Can you work these out from the model? Positions are in its coordinate system, mm. Face numbers are marked on the shaded views. A direction names the side the tool comes from. Give positions to 0.01 mm unless a question says otherwise; leave off trailing zeros. Order: outer loops, then holes, each group sorted by start corner. A loop starts at its lowest first (then second) coordinate and runs counter-clockwise, first axis right, second up. Notation, with made-up numbers: M 63,38.5 L 111,38.5 A33 cw 111,70.5 Z; hole C -28.75,60.25 d3. An arc over 180 degrees is marked long. One line per question, with ' | ' between items. Start each with the question number.
1) Please list where these lines run through material, in increasing order: line 1 along X through (y, z) = (0, 1.25); line 2 along Z through (x, y) = (-3.5, -4); line 3 along Y through (x, z) = (-11.5, -16.5). Write a range as [from, to].
2) For the marked faces 1 and 2, which set-ups out of +Z, -Z, +X, -X, +Y, -Y let a thin tool reach every point of the face, with its end or its side?
3) If we section it at A-A, the plane x = -9: Please give me the cut outline in (y, z).
4) If we section it at B-B, the plane y = 0: Please give me the cut outline in (x, z), plus the area to 3 significant figures.
5) If we section it at C-C, the plane z = -15.25: Please give me the cut outline in (x, y).
6) I'm going to push flat-ended pins straight in: pin 1 Ø1 at (x, y) = (8.5, -4.5) entering from -Z; pin 2 Ø8 at (x, z) = (0, -14.4) entering from -Y. Where does each tip first touch, or does it pass through?
7) If we section it at D-D, the plane x = 0: Please give me the cut outline in (y, z).
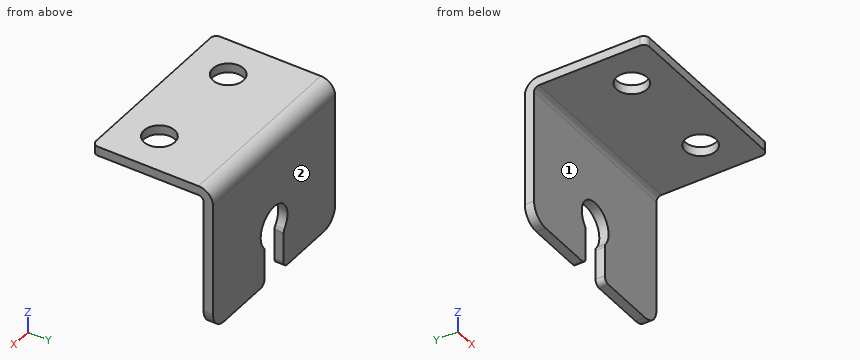
Autodesk Inventor part; units mm, degrees
ref_plane "YZ Plane" through (0, 0, 0) normal (1, 0, 0) x (0, 1, 0)
ref_plane "XZ Plane" through (0, 0, 0) normal (0, 1, 0) x (-1, 0, 0)
ref_plane "XY Plane" through (0, 0, 0) normal (0, 0, 1) x (1, 0, 0)
sketch "Sketch1" plane through (0, 0, 0) normal (0, 0, 1) x (1, 0, 0)
  line L0 (16, -7) -> (-16, -7)
  line L1 (-16, -7) -> (-16, 7)
  line L2 (-16, 7) -> (16, 7)
  line L3 (16, 7) -> (16, -7)
  line L4 (16, -7) -> (-16, 7) construction
  line L5 (-16, -7) -> (16, 7) construction
  line L6 (-9, 0) -> (9, 0) construction
  line L7 (-16, 7) -> (16, 7)
  line L8 (16, 7) -> (16, 12.25)
  line L9 (16, 12.25) -> (-16, 12.25)
  line L10 (-16, 12.25) -> (-16, 7)
  point P0 (0, 0)
  dimension "d126" = 32
  dimension "d127" = 14
  dimension "d128" = 7
  dimension "d129" = 12.25
extrude "Plate4" add sketch "Sketch1" along normal blind 1.6002
fillet "Fillet7" radius 1 2 edges at (16, -7, 0.8001) (-16, -7, 0.8001)
hole "Hole4" at (-9, 0, 0) at (9, 0, 0) direction (0, 0, 1) diameter 5.3 end through all
sketch "Sketch10" plane through (16, 12.25, 0) normal (0, 1, 0) x (-1, 0, 0)
  line L0 (32, 0) -> (0, 0)
  line L1 (0, 0) -> (0, -23.3998)
  line L2 (0, -23.3998) -> (32, -23.3998)
  line L3 (32, -23.3998) -> (32, 0)
edge flange "Flange5" height 25 angle 90 thickness 1.6002 bend radius 0.889 thickness toward (0, 1, 0) relief tear relief width 1.6002 relief depth 0.8001 edges at (0, 12.25, 0) wall of the first edge with corners at (-16, 12.25, 0) (16, 12.25, 0) (16, 12.25, -23.3998) (-16, 12.25, -23.3998)
bend "Bend5"
corner "Corner5"
fillet "Fillet8" radius 3 2 edges at (16, 13.0501, -23.3998) (-16, 13.0501, -23.3998)
sketch "Sketch11" plane through (-16, 13.8502, -0.889) normal (0, 1, 0) x (1, 0, 0)
  arc A0 (32, 19.5108) -> (29, 22.5108) centre (29, 19.5108) ccw
  line L0 (3, 22.5108) -> (29, 22.5108)
  arc A1 (3, 22.5108) -> (0, 19.5108) centre (3, 19.5108) ccw
  line L1 (0, 0) -> (0, 19.5108)
  line L2 (0, 0) -> (32, 0)
  line L3 (32, 19.5108) -> (32, 0)
  circle A2 centre (16, 13.5108) radius 3.5
  line L4 (13.5, 22.5108) -> (18.5, 22.5108)
  line L5 (18.5, 22.5108) -> (18.5, 15.9603)
  line L6 (18.5, 15.9603) -> (13.5, 15.9603)
  line L7 (13.5, 15.9603) -> (13.5, 22.5108)
  point P0 (16, -0.889)
  point P1 (16, 22.5108)
  dimension "d149" = 7
  dimension "d150" = 9
  dimension "d151" = 5
extrude "Extrusion7" cut sketch "Sketch11" against normal through all contours L5 A2 L7 L0 | L6 A2 | A2 L6
fillet "Fillet9" radius 1 2 edges at (-2.5, 13.0501, -16.8493) (2.5, 13.0501, -16.8493)
fillet "Fillet10" radius 1 2 edges at (-2.5, 13.0501, -23.3998) (2.5, 13.0501, -23.3998)
equation "\"d71\" = Thickness"
equation "\"BendReliefWidth\" = Thickness"
equation "\"BendReliefDepth\" = 0.5 * Thickness"
equation "\"CornerReliefSize\" = 4 * Thickness"
equation "\"MinimumRemnant\" = 2 * Thickness"
equation "\"TransitionRadius\" = BendRadius"
equation "\"JacobiRadiusSize\" = BendRadius"
equation "\"GapSize\" = Thickness"
properties part number "Door Stop" material "Aluminum 6061"
Results found:
1) line 1: x = [-16, -11.65], [-6.35, 6.35], [11.65, 16] | line 2: z = [0, 1.6] | line 3: y = [12.25, 13.85]
2) face 1: -Z, +X, -X, -Y | face 2: +Z, -Z, +X, -X, +Y
3) outline: M -7,0 L -2.65,0 L -2.65,1.6 L -7,1.6 Z; M 2.65,0 L 11.36,0 A0.89 cw 12.25,-0.89 L 12.25,-23.4 L 13.85,-23.4 L 13.85,-0.89 A2.49 ccw 11.36,1.6 L 2.65,1.6 Z
4) outline: M -16,0 L -11.65,0 L -11.65,1.6 L -16,1.6 Z; M -6.35,0 L 6.35,0 L 6.35,1.6 L -6.35,1.6 Z; M 11.65,0 L 16,0 L 16,1.6 L 11.65,1.6 Z | area: 34.2 mm²
5) outline: M -16,12.25 L -3.4,12.25 L -3.4,13.85 L -16,13.85 Z; M 3.4,12.25 L 16,12.25 L 16,13.85 L 3.4,13.85 Z
6) pin 1: stops at z = 0 | pin 2: stops at y = 12.25
7) outline: M -7,0 L 11.36,0 A0.89 cw 12.25,-0.89 L 12.25,-10.9 L 13.85,-10.9 L 13.85,-0.89 A2.49 ccw 11.36,1.6 L -7,1.6 Z
